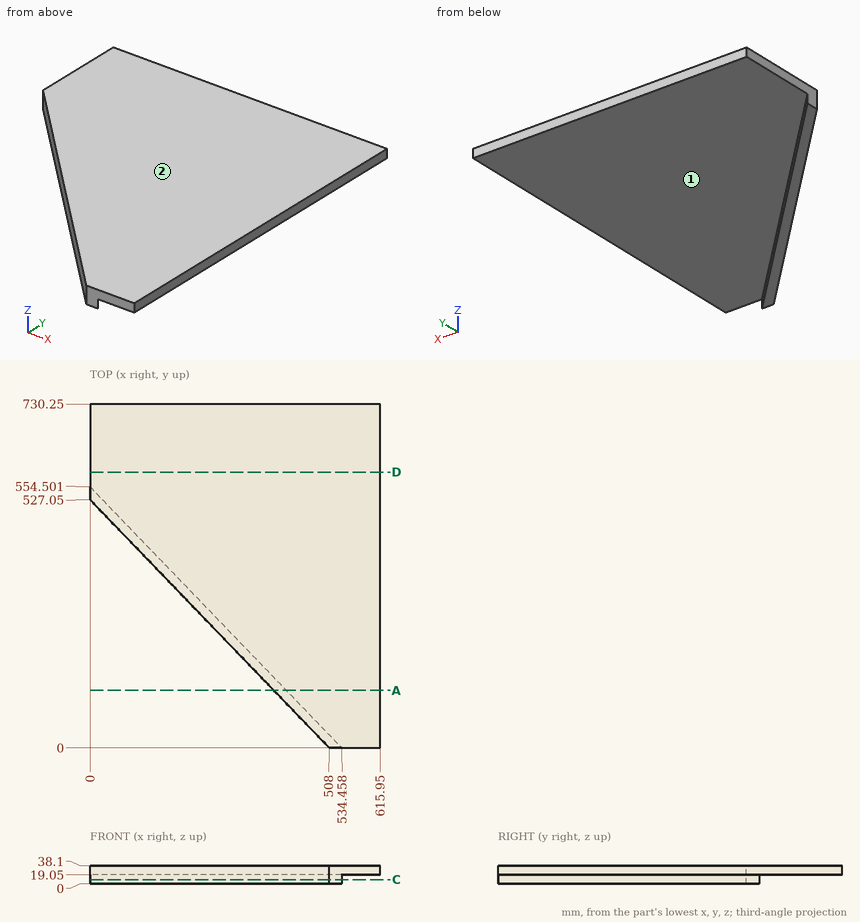
For this review, use the dimensioned drawing (mm, ordinates from the lowest corner) and the shaded views. A direction names the side the tool comes from. Round coordinates to 2 decimals unless told otherwise and drop trailing zeros. Loops run counter-clockwise (first coordinate to the right, second up) from the corner with the lowest first, then second, coordinate; pieces in that order, holes last. Notation, with made-up numbers: (42, -20.75) -> (84, -20.75) arc R31 ccw to (84, 10.25) -> close; hole circle Ø1 at (85.25, 6). An arc over 180 degrees is marked (long way). Write item = value, one per line. Start each with the question number.
Item 1: Take a section at D-D on y = 585.5. Give the boundary of the cut face in (x, z), plus the area to 3 significant figures.
Item 2: For the marked faces 1 and 2, list the 3-axis set-ups (+Z, -Z, +X, -X, +Y, -Y) from which the entire face can be reached by the end or side of a thin tool; tool diameter is ignored.
Item 3: Take a section at A-A on y = 122. Give the boundary of the cut face in (x, z).
Item 4: To check wall thickness, follow L1, parallel to Z at x = 203.5, y = 377.5; L2, parallel to X at y = 80.5, z = 36.5; L3, parallel to Y at x = 332.5, z = 25.5. State the ranges of each line that lie inside material, in increasing order.
Item 5: Take a section at C-C on z = 9. Give the boundary of the cut face in (x, y).
Item 6: Insertion check: pin 1 (8 mm diameter, centred on x = 471.5, z = 8, fed in from +Y); pin 2 (1.5 mm diameter, centred on x = 429, y = 551.5, fed in from -Z); pin 3 (1.5 mm diameter, centred on y = 422.5, z = 30, fed in from -X). Each pin has a flat end and moves straight along its axis. Give the tip position at first contact, or say it passes through.
Result:
q1.outline = (0, 19.05) -> (615.95, 19.05) -> (615.95, 38.1) -> (0, 38.1) -> close
q1.area = 11,700 mm²
q2.face_1 = -Z, +X, +Y
q2.face_2 = +Z, +X, -X, +Y, -Y
q3.outline = (390.41, 0) -> (416.87, 0) -> (416.87, 19.05) -> (615.95, 19.05) -> (615.95, 38.1) -> (390.41, 38.1) -> close
q4.L1 = 19.05 to 38.1
q4.L2 = 430.41 to 615.95
q4.L3 = 182.08 to 730.25
q5.outline = (0, 527.05) -> (508, 0) -> (534.46, 0) -> (0, 554.5) -> close
q6.pin_1 = 69.47
q6.pin_2 = 19.05
q6.pin_3 = 100.05
